Check sheet for the modelled part. Datum: model origin and axes. Units: mm. Round coordinates to 2 decimals unless told otherwise and drop trailing zeros. Loops run counter-clockwise (first coordinate to the right, second up) from the corner with the lowest first, then second, coordinate; pieces in that order, holes last. Notation, with made-up numbers: (-10.5, 71) -> (35.5, 71) arc R15 ccw to (35.5, 79) -> close; hole circle Ø2 at (77, 13). An arc over 180 degrees is marked (long way). One line per item, written item: value. Start each with the question number.
1. Cross-section at B-B on y = 12. Record the cut outline in (x, z) (3 decimals), then the cut area to 3 significant figures.
2. Cross-section at C-C on x = 1.5. Record the cut outline in (y, z) (3 decimals).
3. Cross-section at D-D on z = 2.5. Record the cut outline in (x, y), then the cut area to 3 significant figures.
4. Material ranges on L1, parallel to Z at x = 22, y = 21; L2, parallel to Y at x = -2.5, z = 7.5; L3, parallel to Y at x = -3, z = 4.5, recorded low to high.
5. Go/stop test with flat-tipped pins: pin 1 (12 mm diameter, centred on x = 19.5, y = 3, fed in from +Z); pin 2 (1.5 mm diameter, centred on x = 23, y = 16.5, fed in from +Z); pin 3 (12 mm diameter, centred on x = 5.5, y = 9.5, fed in from -Z). Record where each tip stops, or that it passes through.
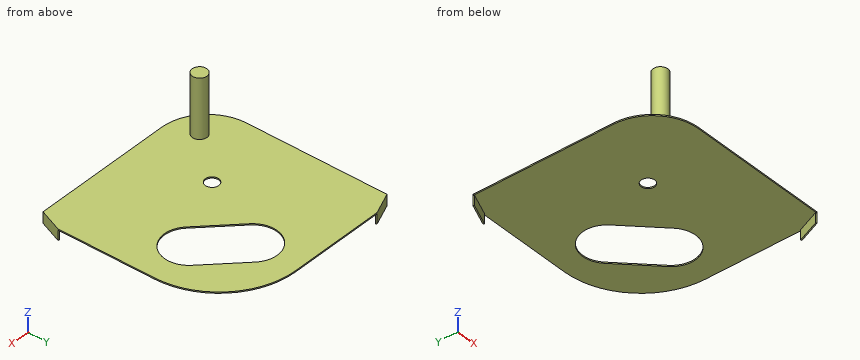
from build123d import *

# Parameters (mm, degrees)
BOSS_EXTRUDE1_DEPTH = 0.254
SKETCH2_R           = 2.032
CUT_EXTRUDE1_DEPTH  = 0.254
SKETCH3_R           = 1.397
CUT_EXTRUDE2_DEPTH  = 0.254
CUT_EXTRUDE3_DEPTH  = 0.254
SKETCH5_R           = 1.524
BOSS_EXTRUDE2_DEPTH = 12.192
BOSS_EXTRUDE3_DEPTH = 2.286
SKETCH8_R           = 2.05178126
BOSS_EXTRUDE4_DEPTH = 0.254
SKETCH9_W           = 2.585879879
SKETCH9_H           = 0.671823721
CUT_EXTRUDE4_DEPTH  = 31.895819587


with BuildPart() as part:
    # Sketch1 → Boss-Extrude1 (new body)
    with BuildSketch(Plane.XY):
        with BuildLine():
            Line((0, -9.525), (29.211998505, -9.525))
            Line((29.211998505, -9.525), (31.115, -4.814906019))
            Line((31.115, -4.814906019), (31.115, 15.24))
            ThreePointArc((31.115, 15.24), (26.465320151, 26.465320151), (15.24, 31.115))
            Line((15.24, 31.115), (-4.814906019, 31.115))
            Line((-4.814906019, 31.115), (-9.525, 29.211998505))
            Line((-9.525, 29.211998505), (-9.525, 0))
            ThreePointArc((-9.525, 0), (-6.735192091, -6.735192091), (0, -9.525))
        make_face()
    extrude(amount=-BOSS_EXTRUDE1_DEPTH)

    # Sketch2 → Cut-Extrude1 (cut)
    with BuildSketch(Plane.XY):
        Circle(SKETCH2_R)
    extrude(amount=-CUT_EXTRUDE1_DEPTH, mode=Mode.SUBTRACT)

    # Sketch3 → Cut-Extrude2 (cut)
    with BuildSketch(Plane.XY):
        with Locations((5.92696904, 5.92696904)):
            Circle(SKETCH3_R)
    extrude(amount=-CUT_EXTRUDE2_DEPTH, mode=Mode.SUBTRACT)

    # Sketch4 → Cut-Extrude3 (cut)
    with BuildSketch(Plane.XY):
        with BuildLine():
            Line((17.601301997, 24.785506894), (24.785506894, 17.601301997))
            ThreePointArc((24.785506894, 17.601301997), (24.785506894, 10.4170971), (17.601301997, 10.4170971))
            Line((17.601301997, 10.4170971), (10.4170971, 17.601301997))
            ThreePointArc((10.4170971, 17.601301997), (10.4170971, 24.785506894), (17.601301997, 24.785506894))
        make_face()
    extrude(amount=-CUT_EXTRUDE3_DEPTH, mode=Mode.SUBTRACT)

    # Sketch5 → Boss-Extrude2 (add)
    with BuildSketch(Plane.XY):
        with Locations((-2.54, -3.81)):
            Circle(SKETCH5_R)
    extrude(amount=BOSS_EXTRUDE2_DEPTH)

    # Sketch7 → Boss-Extrude3 (add)
    with BuildSketch(Plane.XY):
        Polygon((29.211998505, -9.525), (28.976493806, -9.429849925), (30.879495301, -4.719755944), (31.115, -4.814906019), align=None)
        with BuildLine():
            Line((27.708062292, 24.654775211), (27.887667414, 24.834380333))
            ThreePointArc((27.887667414, 24.834380333), (26.465320151, 26.465320151), (24.834380333, 27.887667414))
            Line((24.834380333, 27.887667414), (24.654775211, 27.708062292))
            Line((24.654775211, 27.708062292), (27.708062292, 24.654775211))
        make_face()
        Polygon((-9.525, 29.211998505), (-9.429849925, 28.976493806), (-4.719755944, 30.879495301), (-4.814906019, 31.115), align=None)
    extrude(amount=-BOSS_EXTRUDE3_DEPTH)

    # Sketch8 → Boss-Extrude4 (add)
    with BuildSketch(Plane.XY):
        Circle(SKETCH8_R)
    extrude(amount=-BOSS_EXTRUDE4_DEPTH)

    # Sketch9 → Cut-Extrude4 (cut, through all)
    with BuildSketch(Plane(origin=(-1.526643541, 1.526643541, 0), x_dir=(0, 0, 1), z_dir=(-0.707106781, 0.707106781, 0))):
        with Locations((-1.54693994, 37.362029341)):
            Rectangle(SKETCH9_W, SKETCH9_H)
    extrude(amount=-CUT_EXTRUDE4_DEPTH, mode=Mode.SUBTRACT)


solid = part.part
Taken from the geometry:
1. outline: (-9.525, -0.254) -> (16.018, -0.254) -> (16.018, 0) -> (-9.525, 0) -> close; (25.859, -0.254) -> (31.115, -0.254) -> (31.115, 0) -> (25.859, 0) -> close
1. area: 7.82 mm2
2. outline: (-9.525, -0.254) -> (31.115, -0.254) -> (31.115, 0) -> (-9.525, 0) -> close
3. outline: circle Ø3.05 at (-2.54, -3.81)
3. area: 7.30 mm2
4. L1: z = -0.25 to 0
4. L2: y = -5.33 to -2.29
4. L3: y = -5.26 to -2.36
5. pin 1: stops at z = 0
5. pin 2: passes through
5. pin 3: stops at z = -0.25
